Geometry check sheet. Reference: the model listing, model coordinates, mm. A direction names the side the tool comes from. Round coordinates to 2 decimals unless told otherwise and drop trailing zeros. Loops run counter-clockwise (first coordinate to the right, second up) from the corner with the lowest first, then second, coordinate; pieces in that order, holes last. Notation, with made-up numbers: (-27.75, 72.25) -> (22.25, 72.25) arc R26 ccw to (22.25, 93.25) -> close; hole circle Ø5 at (-33.5, 40). An arc over 180 degrees is marked (long way). Use a Markdown table: item, result. Add a question column.
Q1. Sectioned sample at B-B, the plane z = -4. Enter the section's corners in (x, y), then the cut area to 3 significant figures.
Q2. Gauge pin test, flat ends, axial feed: P1, Ø5.5, axis at x = -26.25, y = 0, coming from the +Z side (3 decimals); P2, Ø1, axis at y = 15, z = -5.5, coming from the -X side; P3, Ø7.5, axis at x = 26.25, y = 0, coming from the -Z side; P4, Ø1.5, axis at y = 1.5, z = -3, coming from the +X side. Record the tip position at first contact, or that the pin passes through.
Q3. Material ranges on L1, parallel to Z at x = -28, y = 3; L2, parallel to X at y = 0, z = -6.5; L3, parallel to X at y = -1, z = 3.5, recorded low to high.
Q4. Release check for a two-part mould opening along X. For faces 4 (the face through (29.3, -1.26, -6.51)), 5 (the face through (-24, 4, 5.5)), 6 (the face through (31.01, -4.62, -6.49)), 7 (the face through (0, 26, 7.5)) record: released by +X, released by -X, zero draft, split by the parting line, or undercut.
Q5. Sectioned sample at C-C, the plane y = 18. Enter the section's corners in (x, z).
Q6. Sectioned sample at D-D, the plane y = 0. Give the number of separate pieces and of enclosed holes in the cut face, then the cut area to 3 significant figures.
Q7. Sectioned sample at A-A, the plane x = -26.25. Enter the section's corners in (y, z).
Q8. Set-up check for faces 1 (the face through (-8.778, 21.356, -0.105)), 2 (the face through (0, 26, -7.5)), 3 (the face through (-32.66, 2.34, 0.08)): record each of +Z, -Z, +X, -X, +Y, -Y from which the full face is reachable in a straight line by a thin tool's end or side.
```python
from build123d import *

# Parameters (mm, degrees)
F1_R        = 3.3
F2_DEPTH    = 7.5
F0_R        = 3.3
F3_DEPTH    = 7.501
F5_DEPTH    = 5.5
F6_T1_DEPTH = 15
F6_T3_DEPTH = 11
F6_T5_DEPTH = 11
F6_T7_DEPTH = 35
F6_T9_DEPTH = 27.7414052161


# Not quite as in the source:
# - a fillet or chamfer that OpenCascade refuses, or shapes differently, is made with other operations: its cross-section is extruded or revolved along the edge and cut away or added
# - a feature names something its author has since deleted; it is built from what else it names


with BuildPart() as f2:
    # F1 (on Top) → F2 (new body, symmetric)
    with BuildSketch(Plane.XY):
        with BuildLine():
            Line((-9.150288423, 22), (0, 22))
            Line((0, 22), (9.150288423, 22))
            Line((9.150288423, 22), (20.6308917204, -2.6202332228))
            ThreePointArc((20.6308917204, -2.6202332228), (24.1294751114, -5.8260942489), (28.8702332228, -5.6191082796))
            Line((28.8702332228, -5.6191082796), (36.8457417487, -1.9000675763))
            Line((36.8457417487, -1.9000675763), (32.5785159717, 7.2510276339))
            Line((32.5785159717, 7.2510276339), (21.0378806259, 32))
            Line((21.0378806259, 32), (0, 32))
            Line((0, 32), (-21.0378806259, 32))
            Line((-21.0378806259, 32), (-32.5785159717, 7.2510276339))
            Line((-32.5785159717, 7.2510276339), (-36.8457417487, -1.9000675763))
            Line((-36.8457417487, -1.9000675763), (-28.8702332228, -5.6191082796))
            ThreePointArc((-28.8702332228, -5.6191082796), (-24.1294751114, -5.8260942489), (-20.6308917204, -2.6202332228))
            Line((-20.6308917204, -2.6202332228), (-9.150288423, 22))
        make_face()
        with Locations((-26.25, 0)):
            Circle(F1_R, mode=Mode.SUBTRACT)
        with Locations((26.25, 0)):
            Circle(F1_R, mode=Mode.SUBTRACT)
    extrude(amount=F2_DEPTH, both=True)

    # F0 (on Top) → F3 (cut, through all)
    with BuildSketch(Plane.XY):
        with Locations((26.25, 0)):
            Circle(F0_R)
        with Locations((-26.25, 0)):
            Circle(F0_R)
    extrude(amount=F3_DEPTH, mode=Mode.SUBTRACT)

    # F4 (on Top) → F5 (cut, symmetric)
    with BuildSketch(Plane.XY):
        Polygon((38.163918051, -9.4593089454), (29.7503979029, 8.5835432382), (11.4094827275, 12.8178771483), (24.044580395, -14.2781772408), align=None)
        Polygon((-29.7503979029, 8.5835432382), (-38.163918051, -9.4593089454), (-24.044580395, -14.2781772408), (-11.4094827275, 12.8178771483), align=None)
    extrude(amount=F5_DEPTH, both=True, mode=Mode.SUBTRACT)

    # F6: fillet of radius 4 on 10 edges, made by hand

    # F6_s2 → F6_t1 (join)
    with BuildSketch(Plane.XY.offset(-7.5)):
        with BuildLine():
            ThreePointArc((6.6020073798, 22), (8.7512058132, 21.3735657833), (10.2272385279, 19.690473047))
            Line((10.2272385279, 19.690473047), (9.150288423, 22))
            Line((9.150288423, 22), (6.6020073798, 22))
        make_face()
        with BuildLine():
            ThreePointArc((-10.2272385279, 19.690473047), (-8.7512058132, 21.3735657833), (-6.6020073798, 22))
            Line((-6.6020073798, 22), (-9.150288423, 22))
            Line((-9.150288423, 22), (-10.2272385279, 19.690473047))
        make_face()
    extrude(amount=F6_T1_DEPTH)

    # F6_s4 → F6_t3 (join)
    with BuildSketch(Plane.XY.offset(-5.5)):
        with BuildLine():
            ThreePointArc((27.8494697672, 9.0224070783), (29.466947114, 8.233510665), (30.574896698, 6.8153998661))
            Line((30.574896698, 6.8153998661), (29.7503979029, 8.5835432382))
            Line((29.7503979029, 8.5835432382), (27.8494697672, 9.0224070783))
        make_face()
        with BuildLine():
            ThreePointArc((-30.574896698, 6.8153998661), (-29.466947114, 8.233510665), (-27.8494697672, 9.0224070783))
            Line((-27.8494697672, 9.0224070783), (-29.7503979029, 8.5835432382))
            Line((-29.7503979029, 8.5835432382), (-30.574896698, 6.8153998661))
        make_face()
    extrude(amount=F6_T3_DEPTH)

    # F6_s6 → F6_t5 (cut)
    with BuildSketch(Plane.XY.offset(-5.5)):
        with BuildLine():
            ThreePointArc((12.8514854221, 14.0627574212), (13.9594350061, 12.6446466223), (15.5769123529, 11.855750209))
            Line((15.5769123529, 11.855750209), (13.6759842172, 12.2946140492))
            Line((13.6759842172, 12.2946140492), (12.8514854221, 14.0627574212))
        make_face()
        with BuildLine():
            ThreePointArc((-12.8514854221, 14.0627574212), (-13.9594350061, 12.6446466223), (-15.5769123529, 11.855750209))
            Line((-15.5769123529, 11.855750209), (-13.6759842172, 12.2946140492))
            Line((-13.6759842172, 12.2946140492), (-12.8514854221, 14.0627574212))
        make_face()
    extrude(amount=F6_T5_DEPTH, mode=Mode.SUBTRACT)

    # F6_s8 → F6_t7 (cut)
    with BuildSketch(Plane.XY.offset(-17.5)):
        with BuildLine():
            ThreePointArc((33.2205106006, -3.5905406233), (35.2888080367, -1.3333900484), (35.1552687018, 1.7251635718))
            Line((35.1552687018, 1.7251635718), (36.8457417487, -1.9000675763))
            Line((36.8457417487, -1.9000675763), (33.2205106006, -3.5905406233))
        make_face()
        with BuildLine():
            ThreePointArc((-35.1552687018, 1.7251635718), (-35.2888080367, -1.3333900484), (-33.2205106006, -3.5905406233))
            Line((-33.2205106006, -3.5905406233), (-36.8457417487, -1.9000675763))
            Line((-36.8457417487, -1.9000675763), (-35.1552687018, 1.7251635718))
        make_face()
    extrude(amount=F6_T7_DEPTH, mode=Mode.SUBTRACT)

    # F6_s10 → F6_t9 (cut)
    with BuildSketch(Plane.XY.offset(-13.8707026081)):
        with BuildLine():
            ThreePointArc((18.4895995827, 32), (20.6387980161, 31.3735657833), (22.1148307308, 29.690473047))
            Line((22.1148307308, 29.690473047), (21.0378806259, 32))
            Line((21.0378806259, 32), (18.4895995827, 32))
        make_face()
        with BuildLine():
            ThreePointArc((-22.1148307308, 29.690473047), (-20.6387980161, 31.3735657833), (-18.4895995827, 32))
            Line((-18.4895995827, 32), (-21.0378806259, 32))
            Line((-21.0378806259, 32), (-22.1148307308, 29.690473047))
        make_face()
    extrude(amount=F6_T9_DEPTH, mode=Mode.SUBTRACT)


solid = f2.part
```
Values:
| question | item | result |
|---|---|---|
| 1 | outline | (-35.16, 1.73) arc R4 ccw to (-34.81, -2.26) -> (-30.57, 6.82) arc R4 cw to (-27.85, 9.02) -> (-15.58, 11.86) arc R4 ccw to (-12.85, 14.06) -> (-10.23, 19.69) arc R4 cw to (-6.6, 22) -> (6.6, 22) arc R4 cw to (10.23, 19.69) -> (12.85, 14.06) arc R4 ccw to (15.58, 11.86) -> (27.85, 9.02) arc R4 cw to (30.57, 6.82) -> (34.81, -2.26) arc R4 ccw to (35.16, 1.73) -> (22.11, 29.69) arc R4 ccw to (18.49, 32) -> (-18.49, 32) arc R4 ccw to (-22.11, 29.69) -> close |
| 1 | area | 900 mm^2 |
| 2 | P1 | through |
| 2 | P2 | x = -29.2 |
| 2 | P3 | z = -7.5 |
| 2 | P4 | x = 35.47 |
| 3 | L1 | -7.5 to -5.5, 5.5 to 7.5 |
| 3 | L2 | -35.53 to -29.55, -22.95 to -19.41, 19.41 to 22.95, 29.55 to 35.53 |
| 3 | L3 | -35.39 to -34.22, 34.22 to 35.39 |
| 4 | face 4 | undercut |
| 4 | face 5 | undercut |
| 4 | face 6 | released by +X |
| 4 | face 7 | zero draft |
| 5 | outline | (-27.57, -7.5) -> (-11.02, -7.5) -> (-11.02, 7.5) -> (-27.57, 7.5) -> close; (11.02, -7.5) -> (27.57, -7.5) -> (27.57, 7.5) -> (11.02, 7.5) -> close |
| 6 | separate pieces | 6 |
| 6 | enclosed holes | 0 |
| 6 | area | 115 mm^2 |
| 7 | outline | (-6.2, -7.5) -> (-3.3, -7.5) -> (-3.3, -5.5) -> (-6.2, -5.5) -> close; (-6.2, 5.5) -> (-3.3, 5.5) -> (-3.3, 7.5) -> (-6.2, 7.5) -> close; (3.3, -7.5) -> (20.82, -7.5) -> (20.82, 7.5) -> (3.3, 7.5) -> (3.3, 5.5) -> (9.39, 5.5) -> (9.39, -5.5) -> (3.3, -5.5) -> close |
| 8 | face 1 | +Z, -Z, -Y |
| 8 | face 2 | -Z, +X, -X, +Y, -Y |
| 8 | face 3 | -Y |
